Input: part model. Units: mm. Frame: model coordinates. Give positions to 0.01 mm unless a question says otherwise; leave off trailing zeros. Loops run counter-clockwise (first coordinate to the right, second up) from the corner with the lowest first, then second, coordinate; pieces in that order, holes last. Notation, with made-up numbers: (20, 15) -> (29, 15) arc R7 ccw to (29, 19) -> close; hole circle Ø7 at (53, 51.25). An arc over 180 degrees is marked (long way). Use CSV: the item, a comma, the result in double quotes.
```python
from build123d import *

# Parameters (mm, degrees)
F1_DEPTH = 615
F3_W     = 30
F3_H     = 6
F4_DEPTH = 54.7497373415
F6_D     = 10
F7_W     = 35
F7_H     = 8
F8_DEPTH = 25


with BuildPart() as f1:
    # F0 (on Front) → F1 (new body, symmetric)
    with BuildSketch(Plane.XZ):
        Polygon((17.6776695297, 0), (24.7487373415, 0), (0, 24.7487373415), (-24.7487373415, 0), (-17.6776695297, 0), (0, 17.6776695297), align=None)
    extrude(amount=F1_DEPTH, both=True)

    # F3 (on offset) → F4 (cut, through all)
    with BuildSketch(Plane.YZ.offset(30)):
        with Locations((590, 21.7487373415)):
            Rectangle(F3_W, F3_H)
        with Locations((-590, 21.7487373415)):
            Rectangle(F3_W, F3_H)
    extrude(amount=-F4_DEPTH, mode=Mode.SUBTRACT)

    # F6 (through all)
    with Locations(Plane.XY.offset(18.7487373415)):
        with Locations((0, -590), (0, 590)):
            Hole(F6_D / 2)

    # F7 (on face) → F8 (cut)
    with BuildSketch(Plane(origin=(12.3743686708, 0, 12.3743686708), x_dir=(0, 1, 0), z_dir=(0.7071067812, 0, 0.7071067812))):
        with Locations((-597.5, -13.5)):
            Rectangle(F7_W, F7_H)
        with Locations((597.5, -13.5)):
            Rectangle(F7_W, F7_H)
    extrude(amount=-F8_DEPTH, mode=Mode.SUBTRACT)


solid = f1.part
```
1) Section query A-A (y = 216.5). Return loops of the section in (x, z), then the cut area to 3 significant figures.
From the geometry:
outline,"(-24.75, 0) -> (-17.68, 0) -> (0, 17.68) -> (17.68, 0) -> (24.75, 0) -> (0, 24.75) -> close"
area,"300 mm^2"
2) Contact query for flat-ended pins moving along their axis: pin 1 (3 mm diameter, centred on x = -19, y = -454.5, fed in from +Z); pin 2 (8 mm diameter, centred on x = 13, z = 21.5, fed in from +Y); pin 3 (6 mm diameter, centred on x = 22, z = 4, fed in from +Y); pin 4 (12 mm diameter, centred on x = -1, y = 397, fed in from -Z). Output: stop coordinate, or through.
From the geometry:
pin 1,"stops at z = 7.25"
pin 2,"passes through"
pin 3,"stops at y = 580"
pin 4,"stops at z = 10.68"
3) Ray query, line 1 (Y direction, x = 2.5, z = 20.5); line 2 (X direction, y = -532, z = 10); line 3 (X direction, y = -590, z = 14). Return the intervals inside material, ascending.
From the geometry:
line 1,"y = -615 to -605, -575 to 575, 605 to 615"
line 2,"x = -14.75 to -7.68, 7.68 to 14.75"
line 3,"x = -10.75 to -5, 5 to 10.75"
